Here's how the part is built. I have some questions about the finished solid (model axes, mm). Face numbers are marked on the shaded views. A direction names the side the tool comes from. Coordinates: 2 decimals unless noted, no trailing zeros. Write each loop counter-clockwise with the first axis right and the second up, starting at its lowest first coordinate (ties: lowest second). Pieces come first, ordered by that corner, then holes.
from build123d import *

# Parameters (mm, degrees)
SKETCH1_R             = 3.175
SKETCH1_R_2           = 2.3622
BOSS_EXTRUDE1_DEPTH   = 3.175
BOSS_EXTRUDE1_2_DEPTH = 3.175
REVOLVE1_OUTLINE_R    = 3.175
REVOLVE1_OUTLINE_R_2  = 2.3622
REVOLVE1_ANGLE        = 180


# Read off the part's stored shape, not the designer's step: Revolve1
with BuildPart() as part:
    # Sketch1 → Boss-Extrude1 (new body)
    with BuildSketch(Plane.XY):
        with Locations((-4.7625, 13.335)):
            Circle(SKETCH1_R)
        with Locations((-4.7625, 13.335)):
            Circle(SKETCH1_R_2, mode=Mode.SUBTRACT)
    extrude(amount=BOSS_EXTRUDE1_DEPTH)



with BuildPart() as body_2:
    # Sketch1 → Boss-Extrude1 2 (new body)
    with BuildSketch(Plane.XY):
        with Locations((-4.7625, 3.81)):
            Circle(SKETCH1_R)
        with Locations((-4.7625, 3.81)):
            Circle(SKETCH1_R_2, mode=Mode.SUBTRACT)
    extrude(amount=BOSS_EXTRUDE1_2_DEPTH)


with BuildPart() as part_1:
    add(part.part)

    add(body_2.part)  # Revolve1 merges body 2
    # Revolve1 outline → Revolve1 (revolve)
    with BuildSketch(Plane(origin=(0, 8.5725, 0), x_dir=(0, -1, 0), z_dir=(0, 0, 1))):
        with Locations((4.7625, -4.7625)):
            Circle(REVOLVE1_OUTLINE_R)
        with Locations((4.7625, -4.7625)):
            Circle(REVOLVE1_OUTLINE_R_2, mode=Mode.SUBTRACT)
    revolve(axis=Axis((0, 8.5725, 0), (1, 0, 0)), revolution_arc=REVOLVE1_ANGLE)


solid = part_1.part
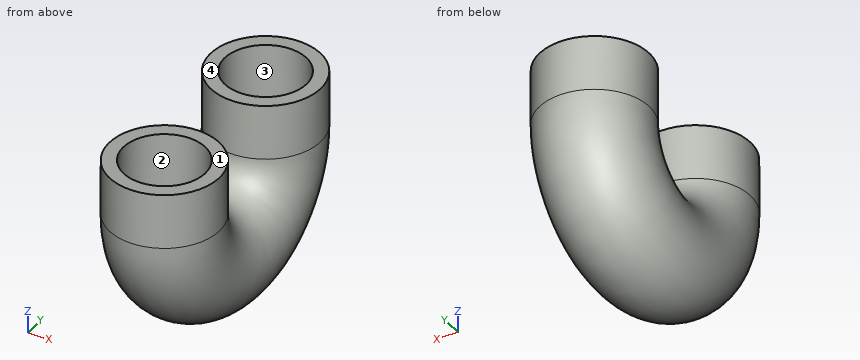
1. If I drill on line 1 (Y direction, x = -4, z = 0); line 2 (X direction, y = 3.81, z = 1.7); line 3 (Y direction, x = -6.25, z = -1.75), over which ranges is the centre line in solid material (lowest first)?
2. I want a section at B-B (z = 0.25). State how many separate pieces and enclosed holes the cut face has, then the cut area to 3 significant figures.
3. I want a section at C-C (x = -3.5). List the corners of the cut face in (y, z) for me (1 decimal), then the cut area to 3 significant figures.
4. Thinking about a two-plate mould opening in Y: for the marked faces 3 and 4, which applies, pulls with the +Y half, pulls with the -Y half, needs draft (parallel to the pull), parting line crosses it, or undercut?
5. On a 3-axis mill with a long thin cutter (end or side, diameter ignored), from which of +Z, -Z, +X, -X, +Y, -Y can I reach the whole of each face in a straight line? I mean the marked faces 1 and 2. Say none if no direction works.
6. I want a section at A-A (x = -6.5). List the corners of the cut face in (y, z) for me (1 decimal), then the cut area to 3 significant figures.
7. For pin 1 Ø2 at (x, y) = (-6, 8.5) entering from +Z; pin 2 Ø2 at (y, z) = (5.5, -6) entering from -X, each with a flat end and sliding along its axis, tell me the tip position at first contact or that it passes through.
Response values:
1. line 1: y = 0.73 to 1.57, 6.05 to 6.89, 10.25 to 11.1, 15.57 to 16.42
1. line 2: x = -7.94 to -7.12, -2.4 to -1.59
1. line 3: y = 1.21 to 2.21, 6.23 to 7.7, 9.45 to 10.92, 14.93 to 15.93
2. separate pieces: 2
2. enclosed holes: 2
2. area: 28.3 mm2
3. outline: (0.9, 0) arc R7.7 ccw to (16.2, 0) - (16.2, 3.2) - (15.3, 3.2) - (15.3, 0) arc R6.8 cw to (1.8, 0) - (1.8, 3.2) - (0.9, 3.2) - close; (5.8, 0) arc R2.8 ccw to (11.3, 0) - (11.3, 3.2) - (10.4, 3.2) - (10.4, 0) arc R1.8 cw to (6.7, 0) - (6.7, 3.2) - (5.8, 3.2) - close
3. area: 39.1 mm2
4. face 3: undercut
4. face 4: needs draft
5. face 1: +Z, +X, -X, +Y, -Y
5. face 2: +Z
6. outline: (1.2, 0) arc R7.4 ccw to (16, 0) - (16, 3.2) - (14.9, 3.2) - (14.9, 0) arc R6.4 cw to (2.2, 0) - (2.2, 3.2) - (1.2, 3.2) - close; (5.4, 0) arc R3.2 ccw to (11.7, 0) - (11.7, 3.2) - (10.7, 3.2) - (10.7, 0) arc R2.1 cw to (6.5, 0) - (6.5, 3.2) - (5.4, 3.2) - close
6. area: 45.1 mm2
7. pin 1: stops at z = -1.38
7. pin 2: stops at x = -7.78
